Here's how the part is built. I have some questions about the finished solid (model axes, mm). Face numbers are marked on the shaded views. A direction names the side the tool comes from. Give positions to 0.01 mm unless a question says otherwise; leave off trailing zeros. Order: outer loops, then holes, each group sorted by start corner. A loop starts at its lowest first (then second) coordinate and runs counter-clockwise, first axis right, second up. Notation, with made-up numbers: (68.25, 18) -> (100.25, 18) arc R13 cw to (100.25, 25) -> close; hole circle Ø3 at (66.25, -32.5). An arc over 180 degrees is marked (long way). Write each question's results on one line, items separated by ' | '. Start each with the question number.
Q1. Imagine slicing it at B-B, the plane x = 6.5. Please give me the cut outline in (y, z).
Q2. Imagine slicing it at C-C, the plane y = -14. Please give me the cut outline in (x, z), then the cut area to 3 significant figures.
Q3. I'm going to push flat-ended pins straight in: pin 1 (5 mm diameter, centred on x = 0.5, z = 13.5, fed in from +Y); pin 2 (1 mm diameter, centred on y = -57, z = -7.5, fed in from +X); pin 3 (1.5 mm diameter, centred on y = -89.5, z = -3.5, fed in from -X); pin 4 (8 mm diameter, centred on x = -3, y = -59, fed in from -Z). Where does each tip first touch, or does it pass through?
Q4. Imagine slicing it at A-A, the plane z = 10. Please give me the cut outline in (x, y), then the cut area to 3 significant figures.
Q5. I need wall thicknesses on line 1 along Y through (x, z) = (0, 16.5); line 2 along X through (y, z) = (-78, 16); line 3 along Y through (x, z) = (0, 29). Which ranges of each line are inside material? Lowest first, please. Write a range as [from, to].
Q6. Thinking about a two-plate mould opening in Y: for the marked faces 1, 2 and 3, which applies, pulls with the +Y half, pulls with the -Y half, needs draft (parallel to the pull), parting line crosses it, or undercut?
Q7. For the marked faces 4 and 5, which set-ups out of +Z, -Z, +X, -X, +Y, -Y let a thin tool reach every point of the face, with its end or its side?
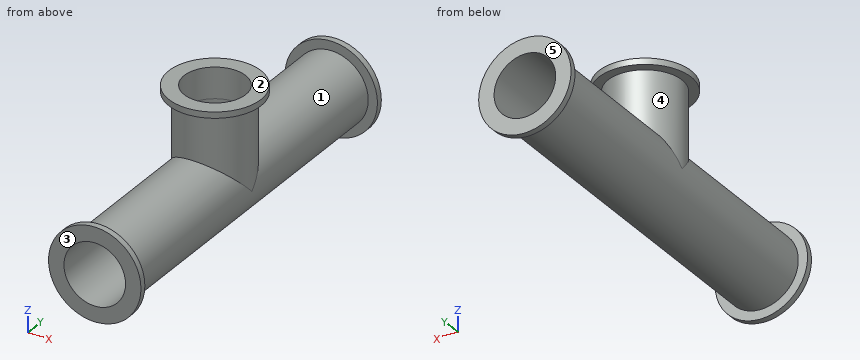
```python
from build123d import *

# Parameters (mm, degrees)
F0_R          = 15.24
F0_R_2        = 12.7
F1_DEPTH      = 157.48
F0_R_3        = 19.05
F2_DEPTH      = 2.54
F3_R          = 19.05
F3_R_2        = 15.24
F4_DEPTH      = 2.54
F6_R          = 15.24
F6_R_2        = 12.7
F7_DEPTH      = 25.4
F7_DEPTH_BACK = 12.7
F8_R          = 19.05
F8_R_2        = 15.24
F9_DEPTH      = 2.54
F10_DEPTH     = 101.6
F8_R_3        = 12.7
F11_DEPTH     = 38.1


with BuildPart() as f1:
    # F0 (on Front) → F1 (new body)
    with BuildSketch(Plane.XZ):
        Circle(F0_R)
        Circle(F0_R_2, mode=Mode.SUBTRACT)
    extrude(amount=F1_DEPTH)

    # F0 (on Front) → F2 (join)
    with BuildSketch(Plane.XZ):
        Circle(F0_R_3)
        Circle(F0_R, mode=Mode.SUBTRACT)
    extrude(amount=F2_DEPTH)

    # F3 (on face) → F4 (join)
    with BuildSketch(Plane.XZ.offset(157.48)):
        Circle(F3_R)
        Circle(F3_R_2, mode=Mode.SUBTRACT)
    extrude(amount=-F4_DEPTH)

    # F6 (on offset) → F7 (join, two sides)
    with BuildSketch(Plane.XY.offset(25.4)) as f7_sk:
        with Locations((0, -78.74)):
            Circle(F6_R)
        with Locations((0, -78.74)):
            Circle(F6_R_2, mode=Mode.SUBTRACT)
    extrude(amount=-F7_DEPTH)
    extrude(f7_sk.sketch, amount=F7_DEPTH_BACK)

    # F8 (on face) → F9 (join)
    with BuildSketch(Plane.XY.offset(38.1)):
        with Locations((0, -78.74)):
            Circle(F8_R)
        with Locations((0, -78.74)):
            Circle(F8_R_2, mode=Mode.SUBTRACT)
    extrude(amount=-F9_DEPTH)

    # F0 (on Front) → F10 (cut)
    with BuildSketch(Plane.XZ):
        Circle(F0_R_2)
    extrude(amount=F10_DEPTH, mode=Mode.SUBTRACT)

    # F8 (on face) → F11 (cut)
    with BuildSketch(Plane.XY.offset(38.1)):
        with Locations((0, -78.74)):
            Circle(F8_R_3)
    extrude(amount=-F11_DEPTH, mode=Mode.SUBTRACT)


solid = f1.part
```
Geometry check:
1) outline: (-157.48, -17.91) -> (-154.94, -17.91) -> (-154.94, -13.78) -> (-2.54, -13.78) -> (-2.54, -17.91) -> (0, -17.91) -> (0, -10.91) -> (-157.48, -10.91) -> close; (-157.48, 10.91) -> (-89.65, 10.91) -> (-89.65, 38.1) -> (-96.65, 38.1) -> (-96.65, 35.56) -> (-92.52, 35.56) -> (-92.52, 13.78) -> (-154.94, 13.78) -> (-154.94, 17.91) -> (-157.48, 17.91) -> close; (-67.83, 10.91) -> (0, 10.91) -> (0, 17.91) -> (-2.54, 17.91) -> (-2.54, 13.78) -> (-64.96, 13.78) -> (-64.96, 35.56) -> (-60.83, 35.56) -> (-60.83, 38.1) -> (-67.83, 38.1) -> close
2) outline: circle Ø30.48 at (0, 0); hole circle Ø25.4 at (0, 0) | area: 223 mm²
3) pin 1: y = 0 | pin 2: x = 13.54 | pin 3: x = -14.99 | pin 4: z = -15.24
4) outline: (-16.21, -157.48) -> (-7.83, -157.48) -> (-7.83, -88.74) arc R12.7 cw to (-7.83, -68.74) -> (-7.83, 0) -> (-16.21, 0) -> (-16.21, -2.54) -> (-11.5, -2.54) -> (-11.5, -68.74) arc R15.24 ccw to (-11.5, -88.74) -> (-11.5, -154.94) -> (-16.21, -154.94) -> close; (7.83, -157.48) -> (16.21, -157.48) -> (16.21, -154.94) -> (11.5, -154.94) -> (11.5, -88.74) arc R15.24 ccw to (11.5, -68.74) -> (11.5, -2.54) -> (16.21, -2.54) -> (16.21, 0) -> (7.83, 0) -> (7.83, -68.74) arc R12.7 cw to (7.83, -88.74) -> close | area: 1,170 mm²
5) line 1: [-157.48, -154.94], [-93.98, -91.44], [-66.04, -63.5], [-2.54, 0] | line 2: [-15.22, -12.68], [12.68, 15.22] | line 3: [-93.98, -91.44], [-66.04, -63.5]
6) face 1: undercut | face 2: needs draft | face 3: pulls with the -Y half
7) face 4: none | face 5: +Z, -Z, +X, -X, +Y
